The listing builds one solid part. Answer for the finished solid, in the listing's coordinates (mm). A direction names the side the tool comes from. Coordinates: 2 decimals unless noted, no trailing zeros. Return JSON: item names as keys, results as strings.
from build123d import *

# Parameters (mm, degrees)
F0_R         = 11.049
F1_DEPTH     = 6.858
F2_DEPTH     = 46.99
F3_DEPTH     = 37.592
F4_DEPTH     = 42.418
F5_DEPTH     = 29.718
F6_DEPTH     = 25.4
F7_T1_DEPTH  = 44.7190403061
F7_T3_DEPTH  = 44.7190403061
F7_T5_DEPTH  = 44.7190403061
F7_T7_DEPTH  = 44.7190403061
F7_T9_DEPTH  = 44.7190403061
F7_T11_DEPTH = 44.7190403061
F7_T14_ANGLE = 117.6067451319
F7_T16_ANGLE = 117.3898443425
F7_T18_ANGLE = 118.1021999746
F7_T20_ANGLE = 118.1021999746
F7_T22_ANGLE = 117.3898443425
F7_T24_ANGLE = 117.6067451319


# Not quite as in the source:
# - a fillet or chamfer that OpenCascade refuses, or shapes differently, is made with other operations: its cross-section is extruded or revolved along the edge and cut away or added


with BuildPart() as f1:
    # F0 (on Top) → F1 (new body)
    with BuildSketch(Plane.XY):
        with BuildLine():
            Line((22.208523276, -31.466120161), (54.2273194105, -31.5911650137))
            Line((54.2273194105, -31.5911650137), (38.3262133623, -3.7995517362))
            ThreePointArc((38.3262133623, -3.7995517362), (18.8280371905, 10.7725526064), (16.14619778, 34.966205418))
            Line((16.14619778, 34.966205418), (0.2450917317, 62.7578186955))
            Line((0.2450917317, 62.7578186955), (-15.8725983546, 35.0912502707))
            ThreePointArc((-15.8725983546, 35.0912502707), (-18.7017871859, 10.8950848293), (-38.354721056, -3.500085257))
            Line((-38.354721056, -3.500085257), (-54.4724111423, -31.1666536818))
            Line((-54.4724111423, -31.1666536818), (-22.4536150077, -31.2916985345))
            ThreePointArc((-22.4536150077, -31.2916985345), (-0.0847964289, -21.7128455258), (22.208523276, -31.466120161))
        make_face()
        Polygon((-41.9885712831, -14.1401743102), (-33.3904459647, -9.2207152943), (-24.8310068248, -14.207180737), (-24.8696930034, -24.1131051956), (-33.4678183218, -29.0325642115), (-42.0272574616, -24.0460987688), align=None, mode=Mode.SUBTRACT)
        Polygon((24.6805966683, -24.3066168019), (24.7192828468, -14.4006923433), (33.3174081652, -9.4812333274), (41.8768473051, -14.4676987701), (41.8381611265, -24.3736232287), (33.2400358081, -29.2930822446), align=None, mode=Mode.SUBTRACT)
        Circle(F0_R, mode=Mode.SUBTRACT)
        Polygon((-8.5839493951, 33.5699382512), (-8.5737367865, 43.4759329869), (0.0102126086, 48.4200859762), (8.5839493951, 43.4582442299), (8.5737367865, 33.5522494943), (-0.0102126086, 28.6080965049), align=None, mode=Mode.SUBTRACT)
        with BuildLine():
            Line((-22.4536150077, -31.2916985345), (22.208523276, -31.466120161))
            ThreePointArc((22.208523276, -31.466120161), (-0.0847964289, -21.7128455258), (-22.4536150077, -31.2916985345))
        make_face()
        with BuildLine():
            ThreePointArc((16.14619778, 34.966205418), (18.8280371905, 10.7725526064), (38.3262133623, -3.7995517362))
            Line((38.3262133623, -3.7995517362), (16.14619778, 34.966205418))
        make_face()
        with BuildLine():
            Line((-15.8725983546, 35.0912502707), (-38.354721056, -3.500085257))
            ThreePointArc((-38.354721056, -3.500085257), (-18.7017871859, 10.8950848293), (-15.8725983546, 35.0912502707))
        make_face()
    extrude(amount=F1_DEPTH)

    # F0 (on Top) → F2 (cut)
    with BuildSketch(Plane.XY):
        with BuildLine():
            Line((-15.8725983546, 35.0912502707), (-38.354721056, -3.500085257))
            ThreePointArc((-38.354721056, -3.500085257), (-18.7017871859, 10.8950848293), (-15.8725983546, 35.0912502707))
        make_face()
    extrude(amount=F2_DEPTH, mode=Mode.SUBTRACT)

    # F0 (on Top) → F3 (cut)
    with BuildSketch(Plane.XY):
        with BuildLine():
            Line((-22.4536150077, -31.2916985345), (22.208523276, -31.466120161))
            ThreePointArc((22.208523276, -31.466120161), (-0.0847964289, -21.7128455258), (-22.4536150077, -31.2916985345))
        make_face()
    extrude(amount=F3_DEPTH, mode=Mode.SUBTRACT)

    # F0 (on Top) → F4 (cut)
    with BuildSketch(Plane.XY):
        with BuildLine():
            ThreePointArc((16.14619778, 34.966205418), (18.8280371905, 10.7725526064), (38.3262133623, -3.7995517362))
            Line((38.3262133623, -3.7995517362), (16.14619778, 34.966205418))
        make_face()
    extrude(amount=F4_DEPTH, mode=Mode.SUBTRACT)

    # F0 (on Top) → F5 (cut)
    with BuildSketch(Plane.XY):
        Circle(F0_R)
    extrude(amount=F5_DEPTH, mode=Mode.SUBTRACT)

    # F0 (on Top) → F6 (cut)
    with BuildSketch(Plane.XY):
        Circle(F0_R)
    extrude(amount=F6_DEPTH, mode=Mode.SUBTRACT)

    # F7: fillet of radius 2.54 on 18 edges, made by hand

    # F7_s2 → F7_t1 (cut)
    with BuildSketch(Plane(origin=(-7.936508422, 13.8712597833, 0), x_dir=(0, 0, 1), z_dir=(-0.4966140739, 0.8679714636, 0))):
        with BuildLine():
            ThreePointArc((0, 28.8391486396), (0.7439487758, 30.6351998638), (2.54, 31.3791486396))
            Line((2.54, 31.3791486396), (0, 31.3791486396))
            Line((0, 31.3791486396), (0, 28.8391486396))
        make_face()
        with BuildLine():
            ThreePointArc((6.858, 28.8391486396), (6.1140512242, 30.6351998638), (4.318, 31.3791486396))
            Line((4.318, 31.3791486396), (6.858, 31.3791486396))
            Line((6.858, 31.3791486396), (6.858, 28.8391486396))
        make_face()
    extrude(amount=F7_T1_DEPTH, mode=Mode.SUBTRACT)

    # F7_s4 → F7_t3 (cut)
    with BuildSketch(Plane(origin=(30.1446132086, -52.6861106484, 0), x_dir=(0, 0, 1), z_dir=(-0.4966140739, 0.8679714636, 0))):
        with BuildLine():
            ThreePointArc((2.54, 31.3791486396), (0.7439487758, 30.6351998638), (0, 28.8391486396))
            Line((0, 28.8391486396), (0, 31.3791486396))
            Line((0, 31.3791486396), (2.54, 31.3791486396))
        make_face()
        with BuildLine():
            ThreePointArc((4.318, 31.3791486396), (6.1140512242, 30.6351998638), (6.858, 28.8391486396))
            Line((6.858, 28.8391486396), (6.858, 31.3791486396))
            Line((6.858, 31.3791486396), (4.318, 31.3791486396))
        make_face()
    extrude(amount=F7_T3_DEPTH, mode=Mode.SUBTRACT)

    # F7_s6 → F7_t5 (cut)
    with BuildSketch(Plane(origin=(15.9811175658, -0.0624119809, 0), x_dir=(0, 0, 1), z_dir=(0.9999923742, -0.0039053279, 0))):
        with BuildLine():
            ThreePointArc((0, 28.8391486396), (0.7439487758, 30.6351998638), (2.54, 31.3791486396))
            Line((2.54, 31.3791486396), (0, 31.3791486396))
            Line((0, 31.3791486396), (0, 28.8391486396))
        make_face()
        with BuildLine():
            ThreePointArc((6.858, 28.8391486396), (6.1140512242, 30.6351998638), (4.318, 31.3791486396))
            Line((4.318, 31.3791486396), (6.858, 31.3791486396))
            Line((6.858, 31.3791486396), (6.858, 28.8391486396))
        make_face()
    extrude(amount=F7_T5_DEPTH, mode=Mode.SUBTRACT)

    # F7_s8 → F7_t7 (cut)
    with BuildSketch(Plane(origin=(-8.0446091438, -13.8088478024, 0), x_dir=(0, 0, 1), z_dir=(-0.5033783003, -0.8640661357, 0))):
        with BuildLine():
            ThreePointArc((0, 28.8391486396), (0.7439487758, 30.6351998638), (2.54, 31.3791486396))
            Line((2.54, 31.3791486396), (0, 31.3791486396))
            Line((0, 31.3791486396), (0, 28.8391486396))
        make_face()
        with BuildLine():
            ThreePointArc((6.858, 28.8391486396), (6.1140512242, 30.6351998638), (4.318, 31.3791486396))
            Line((4.318, 31.3791486396), (6.858, 31.3791486396))
            Line((6.858, 31.3791486396), (6.858, 28.8391486396))
        make_face()
    extrude(amount=F7_T7_DEPTH, mode=Mode.SUBTRACT)

    # F7_s10 → F7_t9 (cut)
    with BuildSketch(Plane(origin=(-60.6998168524, 0.2370544983, 0), x_dir=(0, 0, 1), z_dir=(0.9999923742, -0.0039053279, 0))):
        with BuildLine():
            ThreePointArc((0, 28.8391486396), (0.7439487758, 30.6351998638), (2.54, 31.3791486396))
            Line((2.54, 31.3791486396), (0, 31.3791486396))
            Line((0, 31.3791486396), (0, 28.8391486396))
        make_face()
        with BuildLine():
            ThreePointArc((6.858, 28.8391486396), (6.1140512242, 30.6351998638), (4.318, 31.3791486396))
            Line((4.318, 31.3791486396), (6.858, 31.3791486396))
            Line((6.858, 31.3791486396), (6.858, 28.8391486396))
        make_face()
    extrude(amount=F7_T9_DEPTH, mode=Mode.SUBTRACT)

    # F7_s12 → F7_t11 (cut)
    with BuildSketch(Plane(origin=(30.5552036438, 52.4490561501, 0), x_dir=(0, 0, 1), z_dir=(-0.5033783003, -0.8640661357, 0))):
        with BuildLine():
            ThreePointArc((0, 28.8391486396), (0.7439487758, 30.6351998638), (2.54, 31.3791486396))
            Line((2.54, 31.3791486396), (0, 31.3791486396))
            Line((0, 31.3791486396), (0, 28.8391486396))
        make_face()
        with BuildLine():
            ThreePointArc((6.858, 28.8391486396), (6.1140512242, 30.6351998638), (4.318, 31.3791486396))
            Line((4.318, 31.3791486396), (6.858, 31.3791486396))
            Line((6.858, 31.3791486396), (6.858, 28.8391486396))
        make_face()
    extrude(amount=F7_T11_DEPTH, mode=Mode.SUBTRACT)

    # F7_s13 → F7_t14 (revolve, cut)
    with BuildSketch(Plane(origin=(21.6971694487, 39.0990533159, 0), x_dir=(0, 0, 1), z_dir=(0.4852237348, 0.8743900315, 0))):
        with BuildLine():
            ThreePointArc((0, -6.0457943644), (0.7439487758, -4.2497431402), (2.54, -3.5057943644))
            Line((2.54, -3.5057943644), (0, -3.5057943644))
            Line((0, -3.5057943644), (0, -6.0457943644))
        make_face()
    revolve(axis=Axis((45.3732523459, 25.9605259365, 0), (0, 0, 1)), revolution_arc=F7_T14_ANGLE, mode=Mode.SUBTRACT)

    # F7_s15 → F7_t16 (revolve, cut)
    with BuildSketch(Plane(origin=(23.0875297384, -38.3008650951, 0), x_dir=(0, 0, 1), z_dir=(0.5162541117, -0.8564354571, 0))):
        with BuildLine():
            ThreePointArc((0, -5.9721181992), (0.7439487758, -4.176066975), (2.54, -3.4321181992))
            Line((2.54, -3.4321181992), (0, -3.4321181992))
            Line((0, -3.4321181992), (0, -5.9721181992))
        make_face()
    revolve(axis=Axis((-0.2044107419, -52.3411058879, 0), (0, 0, 1)), revolution_arc=F7_T16_ANGLE, mode=Mode.SUBTRACT)

    # F7_s17 → F7_t18 (revolve, cut)
    with BuildSketch(Plane(origin=(-44.6992655412, -0.5657482073, 0), x_dir=(0, 0, 1), z_dir=(-0.9999199127, -0.0126557538, 0))):
        with BuildLine():
            ThreePointArc((0, -6.2140449518), (0.7439487758, -4.4179937276), (2.54, -3.6740449518))
            Line((2.54, -3.6740449518), (0, -3.6740449518))
            Line((0, -3.6740449518), (0, -6.2140449518))
        make_face()
    revolve(axis=Axis((-45.0385149903, 26.2380507555, 0), (0, 0, 1)), revolution_arc=F7_T18_ANGLE, mode=Mode.SUBTRACT)

    # F7_s19 → F7_t20 (revolve, cut)
    with BuildSketch(Plane(origin=(-21.5544505992, 39.1631213047, 0), x_dir=(0, 0, 1), z_dir=(-0.4821717785, 0.8760766953, 0))):
        with BuildLine():
            ThreePointArc((6.858, 6.2140449518), (6.1140512242, 4.4179937276), (4.318, 3.6740449518))
            Line((4.318, 3.6740449518), (6.858, 3.6740449518))
            Line((6.858, 3.6740449518), (6.858, 6.2140449518))
        make_face()
    revolve(axis=Axis((-45.0385149903, 26.2380507555, 6.858), (0, 0, -1)), revolution_arc=F7_T20_ANGLE, mode=Mode.SUBTRACT)

    # F7_s21 → F7_t22 (revolve, cut)
    with BuildSketch(Plane(origin=(-23.3859780913, -38.1193694225, 0), x_dir=(0, 0, 1), z_dir=(-0.5229276359, -0.8523770807, 0))):
        with BuildLine():
            ThreePointArc((6.858, 5.9721181992), (6.1140512242, 4.176066975), (4.318, 3.4321181992))
            Line((4.318, 3.4321181992), (6.858, 3.4321181992))
            Line((6.858, 3.4321181992), (6.858, 5.9721181992))
        make_face()
    revolve(axis=Axis((-0.2044107419, -52.3411058879, 6.858), (0, 0, -1)), revolution_arc=F7_T22_ANGLE, mode=Mode.SUBTRACT)

    # F7_s23 → F7_t24 (revolve, cut)
    with BuildSketch(Plane(origin=(44.7020643692, -1.1084103144, 0), x_dir=(0, 0, 1), z_dir=(0.9996927331, -0.0247878874, 0))):
        with BuildLine():
            ThreePointArc((4.318, 3.5057943644), (6.1140512242, 4.2497431402), (6.858, 6.0457943644))
            Line((6.858, 6.0457943644), (6.858, 3.5057943644))
            Line((6.858, 3.5057943644), (4.318, 3.5057943644))
        make_face()
    revolve(axis=Axis((45.3732523459, 25.9605259365, 6.858), (0, 0, -1)), revolution_arc=F7_T24_ANGLE, mode=Mode.SUBTRACT)


solid = f1.part
1. For faces 5 (the face through (-29.11, -26.54, 3.38)), 6 (the face through (38, -30.76, 0.72)), 7 (the face through (38, -30.8, 6.1)), 8 (the face through (-7.04, 48.73, 0.72)), determine the directions among +Z, -Z, +X, -X, +Y, -Y from which every point of the face is accessible in a straight line to the end or side of a thin tool.
Answer block:
{"face 5": "+Z, -Z", "face 6": "-Z, -X, -Y", "face 7": "+Z, -X, -Y", "face 8": "-Z, -X, +Y"}
2. Determine the mould class of faces 1 (the face through (46.39, -17.89, 3.42)), 2 (the face through (-29.17, -11.68, 3.38)), 3 (the face through (-7.041, 48.734, 6.134)), 4 (the face through (29.02, -26.835, 3.381)) for opening direction X: pulls with the +X half, pulls with the -X half, needs draft (parallel to the pull), parting line crosses it, or undercut.
Answer block:
{"face 1": "pulls with the +X half", "face 2": "undercut", "face 3": "pulls with the -X half", "face 4": "undercut"}
3. Each of these flat-tipped pins is pushed along its axis until it touches: pin 1 Ø1.5 at (y, z) = (-0.5, 5) entering from -X; pin 2 Ø1 at (x, z) = (-37.5, 3) entering from -Y; pin 3 Ø3 at (y, z) = (49.5, 1.5) entering from +X; pin 4 Ø13.5 at (x, y) = (0, 0) entering from +Z. Where does it stop, or does it pass through?
Answer block:
{"pin 1": "stops at x = -31.71", "pin 2": "stops at y = -31.23", "pin 3": "stops at x = 8.57", "pin 4": "passes through"}
4. Consider line 1 (Y direction, x = 0, z = 4); line 2 (Y direction, x = 4, z = 0.75); line 3 (X direction, y = -15.5, z = 1.25). Determine where each line is inside the solid, lowest interval first. Write a range as from..to.
Answer block:
{"line 1": "y = -21.71..-11.05, 11.05..28.61, 48.41..62.34", "line 2": "y = -21.26..-10.3, 10.3..30.92, 46.11..54.71", "line 3": "x = -44.94..-41.99, -24.84..24.71, 41.87..44.62"}
